Work out the finished part from the listing and answer in its coordinate system (mm). Face numbers are marked on the shaded views. A direction names the side the tool comes from. Coordinates: 2 decimals unless noted, no trailing zeros. Order: outer loops, then holes, each group sorted by start corner. A loop starts at its lowest first (then second) coordinate and runs counter-clockwise, first axis right, second up. Notation, with made-up numbers: M 87.25,53 L 118.25,53 A13 ccw 118.25,73 Z; hole C 21,75 d8. An arc over 180 degrees is marked long. Use a Markdown table: item, result.
from build123d import *

# Parameters (mm, degrees)
F0_W          = 44
F0_H          = 94
F1_DEPTH      = 190
F3_DEPTH      = 25.001
F3_DEPTH_BACK = 25.001
F5_DEPTH      = 25.001
F5_DEPTH_BACK = 25.001


with BuildPart() as f1:
    # F0 (on Right) → F1 (new body)
    with BuildSketch(Plane.YZ):
        with BuildLine():
            Line((22, 50), (-22, 50))
            ThreePointArc((-22, 50), (-24.12132, 49.12132), (-25, 47))
            Line((-25, 47), (-25, -47))
            ThreePointArc((-25, -47), (-24.12132, -49.12132), (-22, -50))
            Line((-22, -50), (22, -50))
            ThreePointArc((22, -50), (24.12132, -49.12132), (25, -47))
            Line((25, -47), (25, 47))
            ThreePointArc((25, 47), (24.12132, 49.12132), (22, 50))
        make_face()
        Rectangle(F0_W, F0_H, mode=Mode.SUBTRACT)
    extrude(amount=F1_DEPTH)

    # F2 (on Front) → F3 (cut, two sides)
    with BuildSketch(Plane.XZ) as f3_sk:
        Polygon((30, -50), (0, 50), (0, -50), align=None)
    extrude(amount=F3_DEPTH, mode=Mode.SUBTRACT)
    extrude(f3_sk.sketch, amount=-F3_DEPTH_BACK, mode=Mode.SUBTRACT)

    # F4 (on Front) → F5 (cut, two sides)
    with BuildSketch(Plane.XZ) as f5_sk:
        with BuildLine():
            Line((159.160798, 50), (40.839202, 50))
            ThreePointArc((40.839202, 50), (100, -20), (159.160798, 50))
        make_face()
    extrude(amount=F5_DEPTH, mode=Mode.SUBTRACT)
    extrude(f5_sk.sketch, amount=-F5_DEPTH_BACK, mode=Mode.SUBTRACT)


solid = f1.part
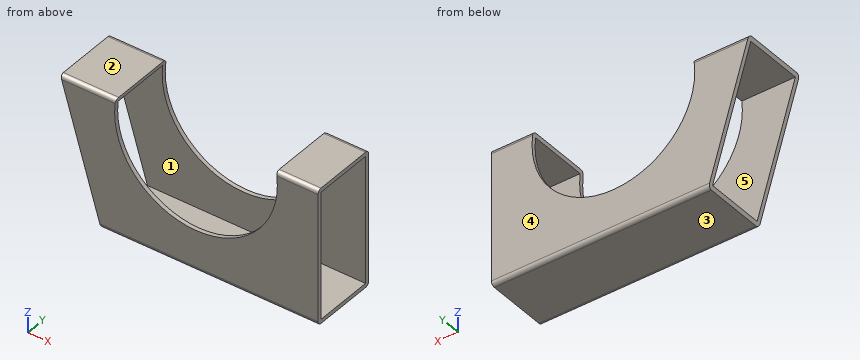
1. For the marked faces 4 and 5, determine the directions among +Z, -Z, +X, -X, +Y, -Y from which every point of the face is accessible in a straight line to the end or side of a thin tool.
Answers below:
| item | result |
|---|---|
| face 4 | +Z, -Z, +X, -X, +Y |
| face 5 | +X, -X |
2. Flat-ended cylindrical pins translate along their axes: P1, Ø10, axis at x = 55.5, y = -11.5, coming from the +Z side; P2, Ø12, axis at x = 24.5, y = 10.5, coming from the -Z side. Find the tip coordinate at first contact, or state that the pin passes through.
Answers below:
| item | result |
|---|---|
| P1 | z = -47 |
| P2 | z = -50 |
3. Find the intervals of material crossed by probe 1 along Y at (x, z) = (43, -18.5); probe 2 along Z at (x, y) = (179, 14); probe 3 along Z at (x, y) = (108.5, 2), in increasing order.
Answers below:
| item | result |
|---|---|
| probe 1 | -25 to -22, 22 to 25 |
| probe 2 | -50 to -47, 47 to 50 |
| probe 3 | -50 to -47 |
4. Section B-B on y = -5 is taken. Determine the outline of the cut face in (x, z), then the cut area to 3 significant figures.
Answers below:
| item | result |
|---|---|
| outline | M 0,50 L 0.9,47 L 40.41,47 A60 cw 40.84,50 Z; M 29.1,-47 L 30,-50 L 190,-50 L 190,-47 Z; M 159.16,50 A60 cw 159.59,47 L 190,47 L 190,50 Z |
| area | 694 mm² |
5. For a pull along Z with two mould halves and no side action, classify the marked faces 1, 2 and 3 as +Z half, -Z half, draft (parallel to the pull), parting line (faces both ways), or undercut.
Answers below:
| item | result |
|---|---|
| face 1 | undercut |
| face 2 | +Z half |
| face 3 | -Z half |
6. Section C-C on x = 18 is taken. Determine the outline of the cut face in (y, z), then the cut area to 3 significant figures.
Answers below:
| item | result |
|---|---|
| outline | M -25,-10 L -22,-10 L -22,47 L 22,47 L 22,-10 L 25,-10 L 25,47 A3 ccw 22,50 L -22,50 A3 ccw -25,47 Z |
| area | 488 mm² |
7. Section A-A on z = 40 is taken. Determine the outline of the cut face in (x, y), then the cut area to 3 significant figures.
Answers below:
| item | result |
|---|---|
| outline | M 3,-25 L 40,-25 L 40,-22 L 3,-22 Z; M 3,22 L 40,22 L 40,25 L 3,25 Z; M 160,-25 L 190,-25 L 190,-22 L 160,-22 Z; M 160,22 L 190,22 L 190,25 L 160,25 Z |
| area | 402 mm² |
8. Section D-D on z = 29.5 is taken. Determine the outline of the cut face in (x, y).
Answers below:
| item | result |
|---|---|
| outline | M 6.15,-25 L 40.93,-25 L 40.93,-22 L 6.15,-22 Z; M 6.15,22 L 40.93,22 L 40.93,25 L 6.15,25 Z; M 159.07,-25 L 190,-25 L 190,-22 L 159.07,-22 Z; M 159.07,22 L 190,22 L 190,25 L 159.07,25 Z |
